Check sheet for the modelled part. Datum: model origin and axes. Units: mm. A direction names the side the tool comes from. Give positions to 0.01 mm unless a question says otherwise; leave off trailing zeros. Write each loop counter-clockwise with the first axis right and the second up, starting at its lowest first coordinate (ties: lowest second). Pieces come first, ordered by that corner, then holes. Notation, with made-up numbers: M 39,-39.5 L 80,-39.5 A22 ccw 80,-25.5 Z; hole C 85,-6 d6. An arc over 180 degrees is marked long. Write item = value, one per line. Start each with the question number.
1) Cross-section at C-C, the plane z = 0. Record the cut outline in (x, y) (3 decimals), plus the area to 3 significant figures.
2) Cross-section at B-B, the plane y = -12.7. Record the cut outline in (x, z) (3 decimals), plus the area to 3 significant figures.
3) Cross-section at A-A, the plane x = 0. Record the cut outline in (y, z) (3 decimals), plus the area to 3 significant figures.
4) Mould release check, pull along Y, two halves, no side actions. Record for faces 1 (the flat face through (133, 38.1, 0)), 2 (the flat face through (58, -6, -3.175)), 3 (the flat face through (58, -38.1, 0)), 4 (the cylindrical face through (0.553, -15.192, -0.044)): released by +Y, released by -Y, zero draft, split by the parting line, or undercut.
5) Access from +Z, -Z, +X, -X, +Y, -Y to the whole of each face (thin tool, end or side, straight path). Record for faces 5 (the flat face through (-19, 25.4, 0)), 6 (the cylindrical face through (136.45, 31.66, 0.69)), 7 (the flat face through (138, 25.4, 0)), 8 (the flat face through (58, -6, 3.175)), 9 (the cylindrical face through (-0.279, 12.703, 0.044)).
6) Scan lines: line 1 along Y through (x, z) = (0, -1.5); line 2 along Y through (x, z) = (-17.5, 2); line 3 along X through (y, z) = (19.5, -1.5). Record each from-to range of solid material in increasing order. Write a range as [from, to].
7) Go/stop test with a flat-tipped pin: pin 1 (1.9 mm diameter, centred on x = 71.5, z = -1, fed in from +Y). Record where the tip stops, or that it passes through.
8) Cross-section at D-D, the plane x = 97.5. Record the cut outline in (y, z) (3 decimals), plus the area to 3 significant figures.
```python
from build123d import *

# Parameters (mm, degrees)
BOSS_EXTRUDE1_DEPTH     = 3.175
F_1_4_20_TAPPED_HOLE1_D = 5.1054
SKETCH4_R               = 3.175
BOSS_EXTRUDE2_DEPTH     = 12.7


with BuildPart() as part:
    # Sketch1 → Boss-Extrude1 (new, symmetric)
    with BuildSketch(Plane.XY):
        with BuildLine():
            Line((-25.4, 25.4), (-12.7, 25.4))
            ThreePointArc((-12.7, 25.4), (0, 12.7), (12.7, 25.4))
            Line((12.7, 25.4), (139.7, 25.4))
            Line((139.7, 25.4), (139.7, -38.1))
            Line((139.7, -38.1), (-25.4, -38.1))
            Line((-25.4, -38.1), (-25.4, 25.4))
        make_face()
    extrude(amount=BOSS_EXTRUDE1_DEPTH, both=True)

    # 1/4-20 Tapped Hole1 (through all)
    with Locations(Plane.XY.offset(3.175)):
        with Locations((0, -12.7)):
            Hole(F_1_4_20_TAPPED_HOLE1_D / 2)

    # Sketch4 → Boss-Extrude2 (add)
    with BuildSketch(Plane(origin=(0, 25.4, 0), x_dir=(1, 0, 0), z_dir=(0, 1, 0))):
        with Locations(Location((133.35, 0, 0), (0, 0, 90))):
            Circle(SKETCH4_R)
    extrude(amount=BOSS_EXTRUDE2_DEPTH)


solid = part.part
```
Reply:
q1.outline = M -25.4,-38.1 L 139.7,-38.1 L 139.7,25.4 L 136.525,25.4 L 136.525,38.1 L 130.175,38.1 L 130.175,25.4 L 12.7,25.4 A12.7 cw -12.7,25.4 L -25.4,25.4 Z; hole C 0,-12.7 d5.105
q1.area = 10,300 mm2
q2.outline = M -25.4,-3.175 L -2.553,-3.175 L -2.553,3.175 L -25.4,3.175 Z; M 2.553,-3.175 L 139.7,-3.175 L 139.7,3.175 L 2.553,3.175 Z
q2.area = 1,020 mm2
q3.outline = M -38.1,-3.175 L -15.253,-3.175 L -15.253,3.175 L -38.1,3.175 Z; M -10.147,-3.175 L 12.7,-3.175 L 12.7,3.175 L -10.147,3.175 Z
q3.area = 290 mm2
q4.face_1 = released by +Y
q4.face_2 = zero draft
q4.face_3 = released by -Y
q4.face_4 = undercut
q5.face_5 = +Z, -Z, -X, +Y
q5.face_6 = +Y
q5.face_7 = +X, +Y
q5.face_8 = +Z, +X, -X, +Y, -Y
q5.face_9 = +Z, -Z, +Y
q6.line_1 = [-38.1, -15.25], [-10.15, 12.7]
q6.line_2 = [-38.1, 25.4]
q6.line_3 = [-25.4, -11.25], [11.25, 139.7]
q7.pin_1 = 25.4
q8.outline = M -38.1,-3.175 L 25.4,-3.175 L 25.4,3.175 L -38.1,3.175 Z
q8.area = 403 mm2
